Solid Edge part; units mm, degrees
sketch "Sketch1" plane through (0, 0, 0) normal (1, 0, 0) x (0, 1, 0)
  line L0 (-14.4105, -33.6582) -> (-54.2057, 6.6977)
  line L1 (-54.2057, 47.6572) -> (-54.2057, 6.6977)
  line L2 (-54.2057, 47.6572) -> (30.6069, 47.6572)
  line L3 (30.6069, 47.6572) -> (30.6069, -58.5082)
  arc A0 (30.6069, -58.5082) -> (-14.4105, -33.6582) centre (50.0394, 29.8961) cw
extrude "Protrusion1" add sketch "Sketch1" against normal blind 15.24
shell "Thinwall_3" thickness 3.81 removed faces 1 at (-15.24, 15.6233, 31.0246)
sketch "Sketch2" plane through (-7.62, -9.7031, 47.6572) normal (0, 0, 1) x (0, -1, 0)
  circle A0 centre (-52.1225, 0) radius 7.62
extrude "Protrusion2" add sketch "Sketch2" against normal up to vertex (106.1654 mm away)
sketch "Sketch3" plane through (-7.62, -9.7031, 47.6572) normal (0, 0, 1) x (0, -1, 0)
  circle A0 centre (-52.1225, 0) radius 5.08
extrude "ExtrudedCutout_4" cut sketch "Sketch3" against normal blind 129.2134
sketch "Sketch4" plane through (-7.62, 30.6069, -5.4255) normal (0, 1, 0) x (0, 0, -1)
  line L0 (-53.0827, 3.9657) -> (-53.0827, 0)
  line L1 (-53.0827, 0) -> (-53.0827, -3.9657)
  line L2 (-53.0827, -3.9657) -> (55.1975, -3.9657)
  line L3 (55.1975, -3.9657) -> (55.1975, 3.9657)
  line L4 (-53.0827, 3.9657) -> (55.1975, 3.9657)
extrude "ExtrudedProtrusion_14" add sketch "Sketch4" along normal blind 6.1628
sketch "Sketch5" plane through (-7.62, -2.0831, 47.6572) normal (0, 0, 1) x (0, 1, 0)
  line L0 (-52.1225, 7.62) -> (-52.1225, -7.62)
  line L1 (-52.1225, 7.62) -> (-42.3273, 7.62)
  arc A0 (-42.3273, 7.62) -> (-52.1226, -7.62) centre (-35.3826, -7.6115) ccw
extrude "ExtrudedCutout_5" cut sketch "Sketch5" against normal blind 61.7549
sketch "Sketch6" plane through (-3.6543, 33.6883, -6.4829) normal (1, 0, 0) x (0, 0, -1)
  line L0 (52.0253, 3.0814) -> (52.0253, -3.0814)
  line L1 (52.0253, -3.0814) -> (54.1401, -3.0814)
  line L2 (54.1401, -3.0814) -> (54.1401, 3.0814)
  line L3 (54.1401, 3.0814) -> (52.0253, 3.0814)
extrude "Cutout1" cut sketch "Sketch6" against normal blind 271.2891
sketch "Sketch7" plane through (0, -11.7994, -5.4255) normal (1, 0, 0) x (0, 1, 0)
  circle A0 centre (-24.3422, 43.2245) radius 4.1013
  circle A1 centre (-24.3422, 14.3323) radius 4.1013
extrude "Cutout2" cut sketch "Sketch7" against normal blind 48.3927
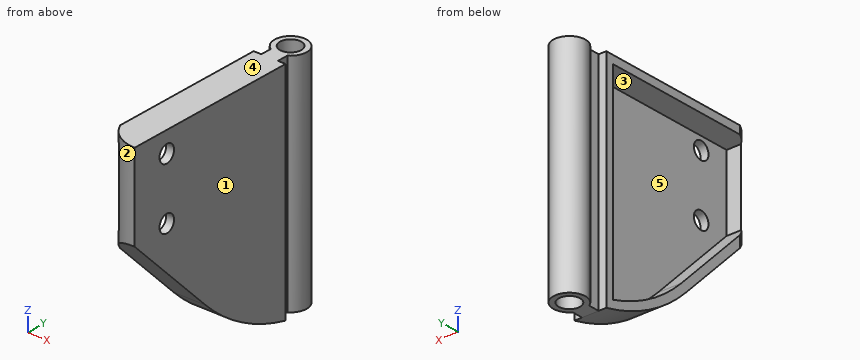
Source: CAD feature listing. Evaluate the final solid. Frame: model axes, mm. Face numbers are marked on the shaded views. A direction names the side the tool comes from. Coordinates: 2 decimals unless noted, no trailing zeros. Order: outer loops, then holes, each group sorted by start corner. A loop starts at its lowest first (then second) coordinate and runs counter-clockwise, first axis right, second up. Notation, with made-up numbers: M 62,-12.75 L 121,-12.75 A24 cw 121,19.25 Z; hole C -6,57.25 d5. An arc over 180 degrees is marked long. Write each question's results on one line, items separated by ' | '. Start each with the question number.
1. Reachability of the marked faces 4 and 5 from +Z, -Z, +X, -X, +Y, -Y: full face, straight path, thin tool, end or side. Return the list, or none.
2. Section C-C, the plane z = -39. Return the cut outline in (x, y).
3. Pin query (flat end, axial travel): pin 1 (6 mm diameter, centred on x = -5, y = 16, fed in from -Z); pin 2 (5.5 mm diameter, centred on x = -12, y = -21.5, fed in from -Z); pin 3 (6 mm diameter, centred on x = -6.5, z = -9.5, fed in from -Y); pin 4 (9 mm diameter, centred on x = -7.62, y = 42.42, fed in from -Z). Return the tip coordinate at first contact, or that it passes through.
4. Section A-A, the plane x = -7.62. Return the cut outline in (y, z), then the cut area to 3 significant figures.
5. Draft query along Y for the marked faces 1, 2 and 3. Return one class per face: +Y half, -Y half, draft (parallel to the pull), parting line (faces both ways), or undercut.
6. Material intervals for L1, parallel to Y at x = -7, z = -16; L2, parallel to Y at x = -4.25, z = 25.5; L3, parallel to X at y = 35, z = -12.5, sorted ascending.
7. Section B-B, the plane y = 42.5. Return the cut outline in (x, z).
8. Section D-D, the plane y = -37. Return the cut outline in (x, z), then the cut area to 3 significant figures.
Solution:
1) face 4: +Z, +X, -X, +Y, -Y | face 5: -X
2) outline: M -15.24,-8.67 L 0,-8.67 L 0,30.61 L -3.65,30.61 L -3.65,35.91 A7.62 ccw long -11.59,35.91 L -11.59,30.61 L -15.24,30.61 L -15.24,26.8 L -3.81,26.8 L -3.81,-2.6 L -15.24,-2.6 Z; hole C -7.62,42.42 d10.16
3) pin 1: z = -55.13 | pin 2: z = -29.26 | pin 3: y = -41.19 | pin 4: through
4) outline: M -52.38,4.84 L -14.41,-33.66 A90.51 ccw 30.61,-58.51 L 37.34,-58.51 L 37.34,47.66 L -52.38,47.66 Z; M 47.5,-58.51 L 50.04,-58.51 L 50.04,47.66 L 47.5,47.66 Z; hole M -50.4,8.26 L -11.7,-30.98 A86.7 ccw 26.8,-53.64 L 26.8,43.85 L -50.4,43.85 Z | area: 2,150 mm²
5) face 1: draft | face 2: -Y half | face 3: undercut
6) L1: -31.82 to -26.47, 26.8 to 37.38, 47.46 to 50.01 | L2: -53.66 to -50.4, 26.8 to 38.62, 46.22 to 49.25 | L3: -11.59 to -3.65
7) outline: M -15.24,-58.51 L -12.7,-58.51 L -12.7,47.66 L -15.24,47.66 Z; M -2.54,-58.51 L 0,-58.51 L 0,47.66 L -2.54,47.66 Z
8) outline: M -15.24,-10.75 L 0,-10.75 L 0,4.9 L -3.81,4.9 L -3.81,-5.32 L -15.24,-5.32 Z; M -15.24,43.85 L -3.81,43.85 L -3.81,41.81 L 0,41.81 L 0,47.66 L -15.24,47.66 Z; M -3.81,12.92 L 0,12.92 L 0,33.79 L -3.81,33.79 Z | area: 267 mm²
